from build123d import *

# Parameters (mm, degrees)
SKETCH1_R            = 227.2
SKETCH1_R_2          = 102
EXTRUDE1_DEPTH       = 2
M4_CLEARANCE_HOLE1_D = 4.3
CIRPATTERN1_COUNT    = 24
M4_CLEARANCE_HOLE2_D = 4.3
M3_CLEARANCE_HOLE1_D = 3.4
CUT_EXTRUDE2_DEPTH   = 3


with BuildPart() as part:
    # Sketch1 → Extrude1 (new body)
    with BuildSketch(Plane.XY):
        Circle(SKETCH1_R)
        Circle(SKETCH1_R_2, mode=Mode.SUBTRACT)
    extrude(amount=EXTRUDE1_DEPTH)

    # M4 Clearance Hole1 (through all)
    with Locations(Plane(origin=(0, 0, 0), x_dir=(-1, 0, 0), z_dir=(0, 0, -1))):
        with Locations((0, 208)):
            m4_clearance_hole1 = Hole(M4_CLEARANCE_HOLE1_D / 2)

    # CirPattern1: M4 Clearance Hole1 ×24 about axis
    cirpattern1_axis = Axis((0, 0, 0), (0, 0, 1))
    for i in range(1, CIRPATTERN1_COUNT):
        add(m4_clearance_hole1.rotate(cirpattern1_axis, i * 360 / CIRPATTERN1_COUNT), mode=Mode.SUBTRACT)

    # M4 Clearance Hole2 (through all)
    with Locations(Plane(origin=(0, 0, 0), x_dir=(-1, 0, 0), z_dir=(0, 0, -1))):
        with Locations((-222, 0), (222, 0)):
            Hole(M4_CLEARANCE_HOLE2_D / 2)

    # M3 Clearance Hole1 (through all)
    with Locations(Plane(origin=(0, 0, 0), x_dir=(-1, 0, 0), z_dir=(0, 0, -1))):
        with Locations((-107.125, 0), (-75.748813935, -75.748813935), (0, -107.125), (75.748813935, -75.748813935), (107.125, 0), (75.748813935, 75.748813935), (0, 107.125), (-75.748813935, 75.748813935)):
            Hole(M3_CLEARANCE_HOLE1_D / 2)

    # Sketch11 → Cut-Extrude2 (cut, through all)
    with BuildSketch(Plane(origin=(0, 0, 0), x_dir=(-1, 0, 0), z_dir=(0, 0, -1))):
        with BuildLine():
            ThreePointArc((222, 6), (216, 0), (222, -6))
            ThreePointArc((222, -6), (225.571486017, -7.531089641), (226.925079563, -11.173552045))
            ThreePointArc((226.925079563, -11.173552045), (227.2, 0), (226.925079563, 11.173552045))
            ThreePointArc((226.925079563, 11.173552045), (225.571486017, 7.531089641), (222, 6))
        make_face()
        with BuildLine():
            ThreePointArc((-222, -6), (-225.571486017, -7.531089641), (-226.925079563, -11.173552045))
            ThreePointArc((-226.925079563, -11.173552045), (-227.2, 0), (-226.925079563, 11.173552045))
            ThreePointArc((-226.925079563, 11.173552045), (-225.571486017, 7.531089641), (-222, 6))
            ThreePointArc((-222, 6), (-216, 0), (-222, -6))
        make_face()
    extrude(amount=-CUT_EXTRUDE2_DEPTH, mode=Mode.SUBTRACT)


solid = part.part
The model under review builds one solid part; all positions refer to its coordinate system, in mm. Round coordinates to 2 decimals unless told otherwise and drop trailing zeros. Order: outer loops, then holes, each group sorted by start corner. A loop starts at its lowest first (then second) coordinate and runs counter-clockwise, first axis right, second up. Notation, with made-up numbers: (-36, 4) -> (-15, 4) arc R9 ccw to (-15, 16) -> close; hole circle Ø6 at (86.25, 60). An arc over 180 degrees is marked (long way). Write item = value, one per line. Start each with the question number.
Item 1: Clearance check with a flat-ended pin moving along its axis: pin 1 Ø1 at (x, z) = (176.5, 1.5) entering from +Y. State where the tip first meets the part, or that it passes through.
Item 2: Consider section C-C on z = 0.7. Count the separate pieces of the cut face and the enclosed holes in it, plus the area to 3 significant figures.
Item 3: Mouldability with a two-part tool opening along X and no side actions: class faces 1 (the face through (-4.84, -227.15, 0.99)), 2 (the face through (-22.112, -99.574, 0.986)), 3 (the face through (-104, 3, 0)) as released by +X, released by -X, zero draft, split by the parting line, or undercut.
Item 4: Consider section A-A on y = -27.5. Write out the cut boundary in (x, z), plus the area to 3 significant figures.
Item 5: Consider section D-D on x = 123. Write out the cut boundary in (y, z), plus the area to 3 significant figures.
Item 6: For line 1 along X through (y, z) = (76.5, 0.1); line 2 along X through (y, z) = (-149, 0.9); line 3 along X through (y, z) = (208, 1.4), list the stretches that pass through material, from the lowest coordinate up.
Item 7: Consider section B-B on y = 191. Write out the cut boundary in (x, z).
Conclusion:
q1.pin_1 = 143.68
q2.separate_pieces = 1
q2.enclosed_holes = 33
q2.area = 129,000 mm2
q3.face_1 = split by the parting line
q3.face_2 = undercut
q3.face_3 = zero draft
q4.outline = (-225.53, 0) -> (-98.22, 0) -> (-98.22, 2) -> (-225.53, 2) -> close; (98.22, 0) -> (225.53, 0) -> (225.53, 2) -> (98.22, 2) -> close
q4.area = 509 mm2
q5.outline = (-191.03, 0) -> (191.03, 0) -> (191.03, 2) -> (-191.03, 2) -> close
q5.area = 764 mm2
q6.line_1 = -213.93 to -77.27, -74.22 to -67.47, 67.47 to 74.22, 77.27 to 213.93
q6.line_2 = -171.52 to -148.04, -146.11 to 146.11, 148.04 to 171.52
q6.line_3 = -91.41 to -2.15, 2.15 to 91.41
q7.outline = (-123.04, 0) -> (123.04, 0) -> (123.04, 2) -> (-123.04, 2) -> close
